Source: CAD feature listing. Evaluate the final solid. Frame: model axes, mm. Round coordinates to 2 decimals unless told otherwise and drop trailing zeros. Write each loop counter-clockwise with the first axis right and the second up, starting at its lowest first coordinate (ties: lowest second). Pieces come first, ordered by that corner, then holes. Notation, with made-up numbers: M -3,64.25 L 56,64.25 A29 cw 56,90.25 Z; hole C 18,-39 d2. An arc over 180 degrees is marked long. Use a Markdown table: item, result.
```python
from build123d import *

# Parameters (mm, degrees)
SKETCH1_W            = 200
SKETCH1_H            = 200
BOSS_EXTRUDE1_DEPTH  = 6.35
SKETCH2_R            = 3.675
CUT_EXTRUDE1_DEPTH   = 142.56384602
M4_CLEARANCE_HOLE1_D = 4.8


with BuildPart() as part:
    # Sketch1 → Boss-Extrude1 (new body)
    with BuildSketch(Plane(origin=(0, 0, 0), x_dir=(1, 0, 0), z_dir=(0, 1, 0))):
        Rectangle(SKETCH1_W, SKETCH1_H)
    extrude(amount=BOSS_EXTRUDE1_DEPTH)

    # Sketch2 → Cut-Extrude1 (cut, through all)
    with BuildSketch(Plane(origin=(0, 6.35, 0), x_dir=(1, 0, 0), z_dir=(0, 1, 0))):
        with Locations(Location((0, 0, 0), (0, 0, 270))):
            Circle(SKETCH2_R)
    extrude(amount=-CUT_EXTRUDE1_DEPTH, mode=Mode.SUBTRACT)

    # M4 Clearance Hole1 (through all)
    with Locations(Plane(origin=(-60.53, 6.35, -60.53), x_dir=(0, 0, 1), z_dir=(0, 1, 0))):
        with Locations((0, 0), (0, 121.06), (121.06, 121.06), (121.06, 0)):
            Hole(M4_CLEARANCE_HOLE1_D / 2)


solid = part.part
```
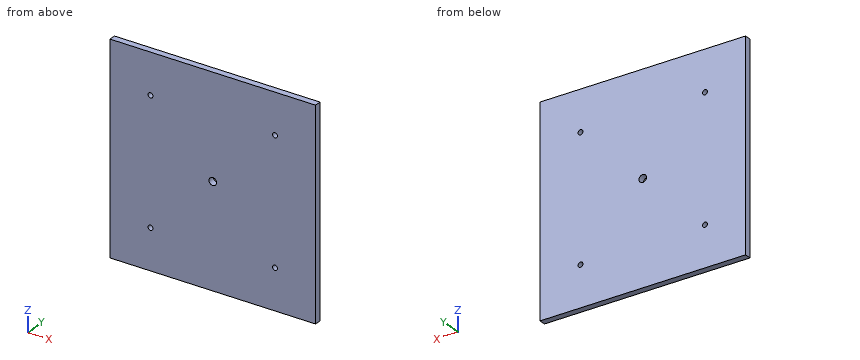
Q1. Section B-B on x = 60.53. Return loops of the section in (y, z).
Results are:
| item | result |
|---|---|
| outline | M 0,-100 L 6.35,-100 L 6.35,-62.93 L 0,-62.93 Z; M 0,-58.13 L 6.35,-58.13 L 6.35,58.13 L 0,58.13 Z; M 0,62.93 L 6.35,62.93 L 6.35,100 L 0,100 Z |
Q2. Line query: L1, parallel to X at y = 5, z = 60.53; L2, parallel to X at y = 1.75, z = 59. Output: solid intervals per line, ascending.
Results are:
| item | result |
|---|---|
| L1 | -100 to -62.93, -58.13 to 58.13, 62.93 to 100 |
| L2 | -100 to -62.38, -58.68 to 58.68, 62.38 to 100 |
Q3. First-contact query: pin 1 Ø6 at (x, z) = (0, 0) entering from +Y (1 decimal). Flat tip, straight axial feed; report the tip coordinate or a pass-through.
Results are:
| item | result |
|---|---|
| pin 1 | through |
Q4. Section D-D on x = 0. Return loops of the section in (y, z) (3 decimals), plus the area to 3 significant figures.
Results are:
| item | result |
|---|---|
| outline | M 0,-100 L 6.35,-100 L 6.35,-3.675 L 0,-3.675 Z; M 0,3.675 L 6.35,3.675 L 6.35,100 L 0,100 Z |
| area | 1,220 mm^2 |
Q5. Section C-C on z = 0. Return loops of the section in (x, y) (3 decimals).
Results are:
| item | result |
|---|---|
| outline | M -100,0 L -3.675,0 L -3.675,6.35 L -100,6.35 Z; M 3.675,0 L 100,0 L 100,6.35 L 3.675,6.35 Z |
Q6. Section A-A on z = 60.53. Return loops of the section in (x, y), plus the area to 3 significant figures.
Results are:
| item | result |
|---|---|
| outline | M -100,0 L -62.93,0 L -62.93,6.35 L -100,6.35 Z; M -58.13,0 L 58.13,0 L 58.13,6.35 L -58.13,6.35 Z; M 62.93,0 L 100,0 L 100,6.35 L 62.93,6.35 Z |
| area | 1,210 mm^2 |
